from build123d import *

# Parameters (mm, degrees)
SKETCH2_W                = 75
SKETCH2_H                = 75
SKETCH2_R                = 21
BOSS_EXTRUDE1_DEPTH      = 4
M4_CLEARANCE_HOLE1_D     = 4.8
M4_CLEARANCE_HOLE1_DEPTH = 55
FILLET1_R                = 6.35


with BuildPart() as part:
    # Sketch1 → Revolve1 (revolve)
    with BuildSketch(Plane.XY, mode=Mode.PRIVATE) as revolve1_sk:
        Polygon((-12, 0), (-29, 0), (-29, 4), (-19, 4), (-19, 55), (-14, 55), (-14, 51.3), (-14.7, 51.3), (-14.7, 50), (-14, 50), (-14, 30), (-12, 30), align=None)
    revolve(revolve1_sk.sketch.rotate(Axis((0, 0, 0), (0, 1, 0)), 270), axis=Axis((0, 0, 0), (0, 1, 0)))

    # Sketch2 → Boss-Extrude1 (add)
    with BuildSketch(Plane(origin=(0, 4, 0), x_dir=(1, 0, 0), z_dir=(0, 1, 0))):
        Rectangle(SKETCH2_W, SKETCH2_H)
        Circle(SKETCH2_R, mode=Mode.SUBTRACT)
    extrude(amount=-BOSS_EXTRUDE1_DEPTH)

    # M4 Clearance Hole1
    with Locations(Plane(origin=(0, 0, 0), x_dir=(-1, 0, 0), z_dir=(0, -1, 0))):
        with Locations((0, 0), (-31.819805153, 31.819805153), (31.819805153, 31.819805153), (31.819805153, -31.819805153), (-31.819805153, -31.819805153)):
            Hole(M4_CLEARANCE_HOLE1_D / 2, depth=M4_CLEARANCE_HOLE1_DEPTH)

    # Fillet1
    fillet1_edges = [part.edges().sort_by_distance(p)[0] for p in [
        (37.5, 2, 37.5),
        (37.5, 2, -37.5),
        (-37.5, 2, -37.5),
        (-37.5, 2, 37.5),
    ]]
    fillet(fillet1_edges, radius=FILLET1_R)


solid = part.part
Geometry: final body of the model. Coordinates: model frame, mm. A direction names the side the tool comes from. Give positions to 0.01 mm unless a question says otherwise; leave off trailing zeros. Write each loop counter-clockwise with the first axis right and the second up, starting at its lowest first coordinate (ties: lowest second). Pieces come first, ordered by that corner, then holes. Notation, with made-up numbers: (50, 55.5) - (106, 55.5) arc R23 cw to (106, 76.5) - close; hole circle Ø9 at (39, 83.5). An arc over 180 degrees is marked (long way). Return JSON: item names as keys, results as strings. Group by question number.
1) Section B-B on x = 0. Return the cut outline in (y, z), plus the area to 3 significant figures.
2) Line query: line 1 (X direction, y = 14, z = 0); line 2 (X direction, y = 51, z = 0); line 3 (Y direction, x = -21, z = 12.5). Output: solid intervals per line, ascending.
3) Section D-D on z = -16.5. Return the cut outline in (x, y).
4) Mould query, pull axis X, two halves, no side actions, for faces 1 (the cylindrical face through (35.59, 1.97, -35.69)), 2 (the flat face through (12, 51.3, 8)), 3 (the flat face through (-9, 0, -9)). Classes: released by +X, released by -X, zero draft, split by the parting line, or undercut.
5) First-contact query: P1, Ø9, axis at x = -0.5, z = 4.5, coming from the +Y side; P2, Ø22.5, axis at x = -13, z = -1.5, coming from the +Y side; P3, Ø6, axis at y = 27.5, z = 14, coming from the +X side; P4, Ø5.5, axis at x = 31.82, z = 31.82, coming from the +Y side. Flat tips, straight axial feed; report the tip coordinate or a pass-through.
6) Section A-A on z = 0. Return the cut outline in (x, y), plus the area to 3 significant figures.
7) Set-up query: faces 4 (the flat face through (37.5, 2, 0)), 5 (the flat face through (8, 50, -12)), 6 (the cylindrical face through (13.67, 53.12, 3.03)). Return all of +Z, -Z, +X, -X, +Y, -Y with unobstructed straight access to the full face (end or side cutting, diameter ignored); none if empty.
8) Section C-C on y = 49. Return the cut outline in (x, z).
Filled in:
{
 "1": {"outline": "(0, -37.5) - (4, -37.5) - (4, -19) - (55, -19) - (55, -14) - (51.3, -14) - (51.3, -14.7) - (50, -14.7) - (50, -14) - (30, -14) - (30, -12) - (0, -12) - close; (0, 12) - (30, 12) - (30, 14) - (50, 14) - (50, 14.7) - (51.3, 14.7) - (51.3, 14) - (55, 14) - (55, 19) - (4, 19) - (4, 37.5) - (0, 37.5) - close", "area": "816 mm^2"},
 "2": {"line 1": "x = -19 to -12, 12 to 19", "line 2": "x = -19 to -14.7, 14.7 to 19", "line 3": "y = 0 to 4"},
 "3": {"outline": "(-37.5, 0) - (37.5, 0) - (37.5, 4) - (9.42, 4) - (9.42, 55) - (-9.42, 55) - (-9.42, 4) - (-37.5, 4) - close"},
 "4": {"face 1": "released by +X", "face 2": "undercut", "face 3": "zero draft"},
 "5": {"P1": "passes through", "P2": "stops at y = 55", "P3": "stops at x = 15.49", "P4": "stops at y = 4"},
 "6": {"outline": "(-37.5, 0) - (-12, 0) - (-12, 30) - (-14, 30) - (-14, 50) - (-14.7, 50) - (-14.7, 51.3) - (-14, 51.3) - (-14, 55) - (-19, 55) - (-19, 4) - (-37.5, 4) - close; (12, 0) - (37.5, 0) - (37.5, 4) - (19, 4) - (19, 55) - (14, 55) - (14, 51.3) - (14.7, 51.3) - (14.7, 50) - (14, 50) - (14, 30) - (12, 30) - close", "area": "816 mm^2"},
 "7": {"face 4": "+Z, -Z, +X, +Y, -Y", "face 5": "none", "face 6": "+Y"},
 "8": {"outline": "circle Ø38 at (0, 0); hole circle Ø28 at (0, 0)"}
}
